Source: CAD feature listing. Evaluate the final solid. Frame: model axes, mm. A direction names the side the tool comes from. Coordinates: 2 decimals unless noted, no trailing zeros. Write each loop counter-clockwise with the first axis right and the second up, starting at its lowest first coordinate (ties: lowest second). Pieces come first, ordered by that corner, then holes. Notation, with made-up numbers: (83.5, 54.25) -> (140.5, 54.25) arc R12 ccw to (140.5, 72.25) -> close; hole circle Ø6 at (65, -1.75). An arc over 180 degrees is marked (long way). Write item = value, one per line.
from build123d import *

# Parameters (mm, degrees)
SKETCH1_W           = 304.8
SKETCH1_H           = 25.4
SKETCH1_R           = 6.35
BOSS_EXTRUDE1_DEPTH = 6.35
BOSS_EXTRUDE2_DEPTH = 6.35
CUT_EXTRUDE1_REACH  = 192.606


with BuildPart() as part:
    # Sketch1 → Boss-Extrude1 (new body)
    with BuildSketch(Plane(origin=(0, 0, 0), x_dir=(1, 0, 0), z_dir=(0, 1, 0))):
        Rectangle(SKETCH1_W, SKETCH1_H)
        with Locations(Location((-139.7, 0, 0), (0, 0, 270))):
            Circle(SKETCH1_R, mode=Mode.SUBTRACT)
        with Locations(Location((139.7, 0, 0), (0, 0, 270))):
            Circle(SKETCH1_R, mode=Mode.SUBTRACT)
    extrude(amount=BOSS_EXTRUDE1_DEPTH)

    # Sketch2 → Boss-Extrude2 (add)
    with BuildSketch(Plane(origin=(0, 6.35, 0), x_dir=(1, 0, 0), z_dir=(0, 1, 0))):
        Polygon((-19.05, -12.7), (-19.05, -114.3), (19.05, -114.3), (19.05, -12.7), (19.05, 25.4), (-19.05, 25.4), align=None)
    extrude(amount=-BOSS_EXTRUDE2_DEPTH)

    # Sketch3 → Cut-Extrude1 (cut, up to next)
    with BuildSketch(Plane(origin=(0, 6.35, 0), x_dir=(1, 0, 0), z_dir=(0, 1, 0)), mode=Mode.PRIVATE) as cut_extrude1_sk1:
        with BuildLine():
            Line((-4.922940563, -95.25), (-4.922940563, 6.35))
            ThreePointArc((-4.922940563, 6.35), (0, 11.272940563), (4.922940563, 6.35))
            Line((4.922940563, 6.35), (4.922940563, -95.25))
            ThreePointArc((4.922940563, -95.25), (0, -100.172940563), (-4.922940563, -95.25))
        make_face()
    cut_extrude1_tool1 = extrude(cut_extrude1_sk1.sketch, amount=-CUT_EXTRUDE1_REACH, mode=Mode.PRIVATE) & part.part
    add(cut_extrude1_tool1.solids().sort_by_distance((0, 6.35, 44.45))[0], mode=Mode.SUBTRACT)


solid = part.part
1) Reachability of faces 1 (the flat face through (85, 3, 12.7)), 2 (the flat face through (-19.05, 3, -19)), 3 (the flat face through (4.923, 3, 44)), 4 (the flat face through (-19.05, 3, 63)), 5 (the flat face through (85, 3, -12.7)) from +Z, -Z, +X, -X, +Y, -Y: full face, straight path, thin tool, end or side. Return the list, or none.
Answer block:
face_1 = +Z, +X, +Y, -Y
face_2 = -Z, -X, +Y, -Y
face_3 = +Y, -Y
face_4 = +Z, -X, +Y, -Y
face_5 = -Z, +X, +Y, -Y
2) Cut plane C-C, the plane y = 1.75. Output: boundary loops of the cut face in (x, z), and give its area (3 significant figures).
Answer block:
outline = (-152.4, -12.7) -> (-19.05, -12.7) -> (-19.05, -25.4) -> (19.05, -25.4) -> (19.05, -12.7) -> (152.4, -12.7) -> (152.4, 12.7) -> (19.05, 12.7) -> (19.05, 114.3) -> (-19.05, 114.3) -> (-19.05, 12.7) -> (-152.4, 12.7) -> close; hole circle Ø12.7 at (-139.7, 0); hole (-4.92, -6.35) arc R4.92 ccw to (4.92, -6.35) -> (4.92, 95.25) arc R4.92 ccw to (-4.92, 95.25) -> close; hole circle Ø12.7 at (139.7, 0)
area = 10,800 mm2
3) Material intervals for probe 1 along X at (y, z) = (1.5, 0); probe 2 along X at (y, z) = (2.5, 33.5); probe 3 along X at (y, z) = (4.5, 104.5), sorted ascending. Write a range as [from, to].
Answer block:
probe_1 = [-152.4, -146.05], [-133.35, -4.92], [4.92, 133.35], [146.05, 152.4]
probe_2 = [-19.05, -4.92], [4.92, 19.05]
probe_3 = [-19.05, 19.05]
4) First-contact query: pin 1 Ø1.9 at (y, z) = (3.5, 71.5) entering from -X; pin 2 Ø11.5 at (x, z) = (139.7, 0) entering from -Y; pin 3 Ø1.5 at (x, y) = (121.5, 5) entering from +Z; pin 4 Ø14.5 at (x, z) = (-139.7, 0) entering from -Y. Flat tips, straight axial feed; report the tip coordinate or a pass-through.
Answer block:
pin_1 = -19.05
pin_2 = through
pin_3 = 12.7
pin_4 = 0
5) Cut plane A-A, the plane z = 0. Output: boundary loops of the cut face in (x, y).
Answer block:
outline = (-152.4, 0) -> (-146.05, 0) -> (-146.05, 6.35) -> (-152.4, 6.35) -> close; (-133.35, 0) -> (-4.92, 0) -> (-4.92, 6.35) -> (-133.35, 6.35) -> close; (4.92, 0) -> (133.35, 0) -> (133.35, 6.35) -> (4.92, 6.35) -> close; (146.05, 0) -> (152.4, 0) -> (152.4, 6.35) -> (146.05, 6.35) -> close
6) Pull-direction query (X, two-part tool) for faces 6 (the flat face through (-152.4, 3, 0)), 7 (the flat face through (-87, 3, 12.7)), 8 (the flat face through (-4.923, 3, 45)); classes: +X half, -X half, draft (parallel to the pull), parting line (faces both ways), or undercut.
Answer block:
face_6 = -X half
face_7 = draft
face_8 = undercut
7) Cut plane D-D, the plane z = 59.5. Output: boundary loops of the cut face in (x, y), and give its area (3 significant figures).
Answer block:
outline = (-19.05, 0) -> (-4.92, 0) -> (-4.92, 6.35) -> (-19.05, 6.35) -> close; (4.92, 0) -> (19.05, 0) -> (19.05, 6.35) -> (4.92, 6.35) -> close
area = 179 mm2
8) Cut plane B-B, the plane x = 139.7. Output: boundary loops of the cut face in (y, z), and give its area (3 significant figures).
Answer block:
outline = (0, -12.7) -> (6.35, -12.7) -> (6.35, -6.35) -> (0, -6.35) -> close; (0, 6.35) -> (6.35, 6.35) -> (6.35, 12.7) -> (0, 12.7) -> close
area = 80.6 mm2
